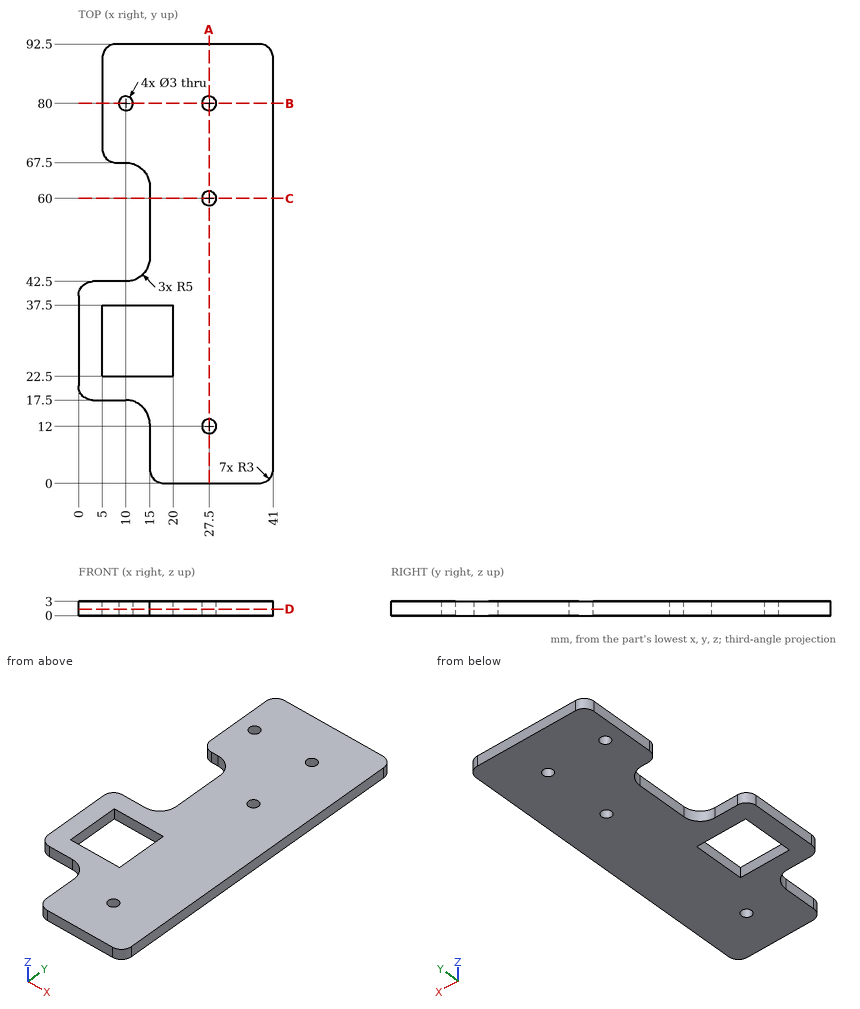
Input: dimensioned drawing with shaded views. Units: mm. Origin: part minimum x, y, z. Coordinates: 2 decimals unless noted, no trailing zeros. Write each loop counter-clockwise with the first axis right and the second up, starting at its lowest first coordinate (ties: lowest second). Pieces come first, ordered by that corner, then holes. Notation, with made-up numbers: M -16.5,71 L 14.5,71 A17 cw 14.5,103 Z; hole C 71.5,83.25 d7. An arc over 180 degrees is marked long. Answer as a JSON object with one key per item and string values. Group by question number.
(1) Contact query for flat-ended pins moving along their axis: P1, Ø1.5, axis at x = 9.5, z = 1, coming from the -Y side; P2, Ø1.5, axis at y = 43, z = 1.5, coming from the -X side; P3, Ø2.5, axis at x = 10, y = 80, coming from the -Z side; P4, Ø1.5, axis at y = 7.5, z = 2, coming from the -X side. Output: stop coordinate, or through.
(2) Section C-C on y = 60. Output: boundary loops of the cut face in (x, z), plus the area to 3 significant figures.
(3) Ray query, line 1 along Y through (x, z) = (10, 1.7); line 2 along Y through (x, z) = (27.5, 1.3); line 3 along X through (y, z) = (80, 2.2). Return the intervals inside material, ascending. Write a range as [from, to].
(4) Section B-B on y = 80. Output: boundary loops of the cut face in (x, z), plus the area to 3 significant figures.
(5) Section D-D on z = 1.35. Output: boundary loops of the cut face in (x, y), plus the area to 3 significant figures.
(6) Section A-A on x = 27.5. Output: boundary loops of the cut face in (y, z).
Result set:
{
 "1": {"P1": "stops at y = 17.49", "P2": "stops at x = 1.8", "P3": "passes through", "P4": "stops at x = 15"},
 "2": {"outline": "M 15,0 L 26,0 L 26,3 L 15,3 Z; M 29,0 L 41,0 L 41,3 L 29,3 Z", "area": "69.0 mm2"},
 "3": {"line 1": "y = [17.5, 22.5], [37.5, 42.5], [67.5, 78.5], [81.5, 92.5]", "line 2": "y = [0, 10.5], [13.5, 58.5], [61.5, 78.5], [81.5, 92.5]", "line 3": "x = [5, 8.5], [11.5, 26], [29, 41]"},
 "4": {"outline": "M 5,0 L 8.5,0 L 8.5,3 L 5,3 Z; M 11.5,0 L 26,0 L 26,3 L 11.5,3 Z; M 29,0 L 41,0 L 41,3 L 29,3 Z", "area": "90.0 mm2"},
 "5": {"outline": "M 0,20.5 A3 ccw 3,17.5 L 10,17.5 A5 cw 15,12.5 L 15,3 A3 ccw 18,0 L 38,0 A3 ccw 41,3 L 41,89.5 A3 ccw 38,92.5 L 8,92.5 A3 ccw 5,89.5 L 5,70.5 A3 ccw 8,67.5 L 10,67.5 A5 cw 15,62.5 L 15,47.5 A5 cw 10,42.5 L 3,42.5 A3 ccw 0,39.5 Z; hole M 5,22.5 L 20,22.5 L 20,37.5 L 5,37.5 Z; hole C 10,80 d3; hole C 27.5,12 d3; hole C 27.5,60 d3; hole C 27.5,80 d3", "area": "2,780 mm2"},
 "6": {"outline": "M 0,0 L 10.5,0 L 10.5,3 L 0,3 Z; M 13.5,0 L 58.5,0 L 58.5,3 L 13.5,3 Z; M 61.5,0 L 78.5,0 L 78.5,3 L 61.5,3 Z; M 81.5,0 L 92.5,0 L 92.5,3 L 81.5,3 Z"}
}
